Check sheet for the modelled part. Datum: model origin and axes. Units: mm. A direction names the side the tool comes from. Give positions to 0.01 mm unless a question says otherwise; leave off trailing zeros. Loops run counter-clockwise (first coordinate to the right, second up) from the corner with the lowest first, then second, coordinate; pieces in that order, holes last. Notation, with made-up numbers: (56, -3) - (114, -3) arc R25 ccw to (114, 29) - close; hole circle Ø9 at (82, 73). An arc over 180 degrees is marked (long way). Use one line per item in the form item = value.
from build123d import *

# Parameters (mm, degrees)
BOSS_EXTRUDE1_DEPTH     = 12.2
SKETCH4_W               = 33
SKETCH4_H               = 1.5
BOSS_EXTRUDE2_DEPTH     = 12.2
SKETCH6_R               = 1.03
CUT_EXTRUDE1_DEPTH      = 5.83
CUT_EXTRUDE1_DEPTH_BACK = 18
SKETCH7_R               = 1.03
CUT_EXTRUDE2_DEPTH      = 5.83
CUT_EXTRUDE2_DEPTH_BACK = 18
SKETCH9_R               = 6
BOSS_EXTRUDE3_DEPTH     = 8.74
SKETCH11_R              = 1.16
BOSS_EXTRUDE4_DEPTH     = 8.74
SKETCH13_W              = 5.4
SKETCH13_H              = 5.45
BOSS_EXTRUDE5_DEPTH     = 7.96
SKETCH14_R              = 2.345
BOSS_EXTRUDE6_DEPTH     = 11.51
SKETCH15_R              = 0.635
CUT_EXTRUDE3_DEPTH      = 3.13
BOSS_EXTRUDE7_START     = 0.8
SKETCH17_R              = 3.355
BOSS_EXTRUDE7_DEPTH     = 3.13
SKETCH18_R              = 0.5
BOSS_EXTRUDE8_DEPTH     = 3.13


with BuildPart() as part:
    # Sketch1 → Boss-Extrude1 (new body)
    with BuildSketch(Plane.XY):
        Polygon((19.12, 0), (23.06, 3.94), (23.06, 21.83), (0, 21.83), (0, 0), align=None)
    extrude(amount=-BOSS_EXTRUDE1_DEPTH)



with BuildPart() as body_2:
    # Sketch4 → Boss-Extrude2 (new body)
    with BuildSketch(Plane.XY):
        with Locations((11.517097498, 16.2852801)):
            Rectangle(SKETCH4_W, SKETCH4_H)
    extrude(amount=-BOSS_EXTRUDE2_DEPTH)

    # Sketch6 → Cut-Extrude1 (cut, two sides)
    with BuildSketch(Plane(origin=(0, 17, 0), x_dir=(1, 0, 0), z_dir=(0, 1, 0))) as cut_extrude1_sk:
        with Locations((-3.31, 6.1)):
            Circle(SKETCH6_R)
    extrude(amount=CUT_EXTRUDE1_DEPTH, mode=Mode.SUBTRACT)
    extrude(cut_extrude1_sk.sketch, amount=-CUT_EXTRUDE1_DEPTH_BACK, mode=Mode.SUBTRACT)

    # Sketch7 → Cut-Extrude2 (cut, two sides)
    with BuildSketch(Plane(origin=(0, 17, 0), x_dir=(1, 0, 0), z_dir=(0, 1, 0))) as cut_extrude2_sk:
        with Locations((26.38, 6.1)):
            Circle(SKETCH7_R)
    extrude(amount=CUT_EXTRUDE2_DEPTH, mode=Mode.SUBTRACT)
    extrude(cut_extrude2_sk.sketch, amount=-CUT_EXTRUDE2_DEPTH_BACK, mode=Mode.SUBTRACT)


with BuildPart() as part_1:
    add(part.part)

    add(body_2.part)  # Boss-Extrude3 merges body 2
    # Sketch9 → Boss-Extrude3 (add)
    with BuildSketch(Plane(origin=(0, 17, 0), x_dir=(1, 0, 0), z_dir=(0, 1, 0))):
        with Locations((17.06, 6.1)):
            Circle(SKETCH9_R)
    extrude(amount=BOSS_EXTRUDE3_DEPTH)

    # Sketch11 → Boss-Extrude4 (add)
    with BuildSketch(Plane(origin=(0, 17, 0), x_dir=(1, 0, 0), z_dir=(0, 1, 0))):
        with Locations((11.06, 6.1)):
            Circle(SKETCH11_R)
    extrude(amount=BOSS_EXTRUDE4_DEPTH)

    # Sketch13 → Boss-Extrude5 (add)
    with BuildSketch(Plane(origin=(0, 17, 0), x_dir=(1, 0, 0), z_dir=(0, 1, 0))):
        with Locations((11.06, 6.1)):
            Rectangle(SKETCH13_W, SKETCH13_H)
    extrude(amount=BOSS_EXTRUDE5_DEPTH)

    # Sketch14 → Boss-Extrude6 (add)
    with BuildSketch(Plane(origin=(0, 17, 0), x_dir=(1, 0, 0), z_dir=(0, 1, 0))):
        with Locations((17.06, 6.1)):
            Circle(SKETCH14_R)
    extrude(amount=BOSS_EXTRUDE6_DEPTH)

    # Sketch15 → Cut-Extrude3 (cut)
    with BuildSketch(Plane(origin=(0, 28.51, 0), x_dir=(1, 0, 0), z_dir=(0, 1, 0))):
        with Locations((17.06, 6.1)):
            Circle(SKETCH15_R)
    extrude(amount=-CUT_EXTRUDE3_DEPTH, mode=Mode.SUBTRACT)

    # Sketch17 → Boss-Extrude7 (add)
    with BuildSketch(Plane(origin=(0, 28.51, 0), x_dir=(1, 0, 0), z_dir=(0, 1, 0)).offset(BOSS_EXTRUDE7_START)):
        with Locations((17.06, 6.1)):
            Circle(SKETCH17_R)
    extrude(amount=-BOSS_EXTRUDE7_DEPTH)

    # Sketch18 → Boss-Extrude8 (add)
    with BuildSketch(Plane(origin=(9.56, -9.56, 0), x_dir=(0, 0, -1), z_dir=(0.707106781, -0.707106781, 0))):
        with Locations((5.09, 18.386997448)):
            Circle(SKETCH18_R)
        with Locations((6.1, 18.386997448)):
            Circle(SKETCH18_R)
        with Locations((7.11, 18.386997448)):
            Circle(SKETCH18_R)
    extrude(amount=BOSS_EXTRUDE8_DEPTH)


solid = part_1.part
Item 1: Thickness scan on L1, parallel to X at y = 16.65, z = -6.1; L2, parallel to Z at x = 26.38, y = 16.35; L3, parallel to Z at x = 17.06, y = 25.8 (3 decimals). Record the ranges inside material, lowest first.
Answer block:
L1 = -4.98 to -4.34, -2.28 to 25.35, 27.41 to 28.02
L2 = -12.2 to -7.13, -5.07 to 0
L3 = -8.445 to -6.735, -5.465 to -3.755
Item 2: Section check A-A on x = -3.31. Record the boundary of the cut face in (y, z).
Answer block:
outline = (15.54, -12.2) - (17.04, -12.2) - (17.04, -7.13) - (15.54, -7.13) - close; (15.54, -5.07) - (17.04, -5.07) - (17.04, 0) - (15.54, 0) - close
Item 3: Gauge pin test, flat ends, axial feed: P1, Ø2.5, axis at x = 26.38, z = -6.1, coming from the +Y side; P2, Ø2, axis at y = 11, z = -4.5, coming from the +X side; P3, Ø3, axis at x = 17, y = 10, coming from the +Z side; P4, Ø2.5, axis at y = 23, z = -6, coming from the -X side. Record the tip position at first contact, or that the pin passes through.
Answer block:
P1 = 17.04
P2 = 23.06
P3 = 0
P4 = 0
Item 4: Section check D-D on y = 4.5. Record the boundary of the cut face in (x, z).
Answer block:
outline = (0, -12.2) - (23.06, -12.2) - (23.06, 0) - (0, 0) - close
Item 5: Access from +Z, -Z, +X, -X, +Y, -Y to the whole of each face (thin tool, end or side, straight path). Record for faces 5 (the face through (-2, 17.035, -6)), 6 (the face through (10, 23, -8.825)), 7 (the face through (23.055, 23.758, -5.852)), 8 (the face through (-2, 15.535, -6)).
Answer block:
face_5 = +Z, -Z, -X, +Y
face_6 = -Z, -X, +Y
face_7 = +Y
face_8 = +Z, -Z, -X, -Y
Item 6: Section check C-C on z = -1. Record the boundary of the cut face in (x, y), then the cut area to 3 significant figures.
Answer block:
outline = (-4.98, 15.54) - (0, 15.54) - (0, 0) - (19.12, 0) - (23.06, 3.94) - (23.06, 15.54) - (28.02, 15.54) - (28.02, 17.04) - (23.06, 17.04) - (23.06, 21.83) - (20.22, 21.83) - (20.22, 25.74) - (13.9, 25.74) - (13.9, 21.83) - (0, 21.83) - (0, 17.04) - (-4.98, 17.04) - close
area = 535 mm2
Item 7: Section check B-B on x = 17.06. Record the boundary of the cut face in (y, z) (3 decimals), then the cut area to 3 significant figures.
Answer block:
outline = (0, -12.2) - (21.83, -12.2) - (21.83, -12.1) - (25.74, -12.1) - (25.74, -8.445) - (26.18, -8.445) - (26.18, -9.455) - (29.31, -9.455) - (29.31, -2.745) - (26.18, -2.745) - (26.18, -3.755) - (25.74, -3.755) - (25.74, -0.1) - (21.83, -0.1) - (21.83, 0) - (0, 0) - close; hole (25.38, -6.735) - (26.18, -6.735) - (26.18, -5.465) - (25.38, -5.465) - close
area = 335 mm2
Item 8: Mould release check, pull along X, two halves, no side actions. Record for faces 1 (the face through (16.98, 25.79, -6.73)), 2 (the face through (25, 17.035, -6)), 3 (the face through (23.06, 19, -6)), 4 (the face through (23.95, 2.65, -5.36)): released by +X, released by -X, zero draft, split by the parting line, or undercut.
Answer block:
face_1 = undercut
face_2 = zero draft
face_3 = released by +X
face_4 = undercut
